```python
from build123d import *

# Parameters (mm, degrees)
BOSS_EXTRUDE1_START = -3
SKETCH2_R           = 9.461289508
BOSS_EXTRUDE1_DEPTH = 3
SKETCH3_R           = 2.54
BOSS_EXTRUDE2_DEPTH = 6
SKETCH4_R           = 2.54
CUT_EXTRUDE1_DEPTH  = 3


with BuildPart() as part:
    # Sketch1 → Revolve1 (revolve)
    with BuildSketch(Plane.XY, mode=Mode.PRIVATE) as revolve1_sk:
        with BuildLine():
            Line((-3, 3), (-3, 0))
            Line((-3, 0), (3, 0))
            ThreePointArc((3, 0), (3.464967985, 1.122532015), (4.5875, 1.5875))
            Line((4.5875, 1.5875), (3, 3))
            Line((3, 3), (0, 3))
            Line((0, 3), (-3, 3))
        make_face()
    revolve(revolve1_sk.sketch.rotate(Axis((-35.1, 18.916479231, 0), (0, -1, 0)), 180), axis=Axis((-35.1, 18.916479231, 0), (0, -1, 0)))

    # Sketch2 → Boss-Extrude1 (add)
    with BuildSketch(Plane(origin=(0, 3, 0), x_dir=(1, 0, 0), z_dir=(0, 1, 0)).offset(BOSS_EXTRUDE1_START)):
        with BuildLine():
            Line((-45.417440708, 11.981122365), (-56.04641595, 24.324014037))
            ThreePointArc((-56.04641595, 24.324014037), (-51.15, 27.799415461), (-45.692006103, 30.302135349))
            Line((-45.692006103, 30.302135349), (-40.31723598, 14.925726938))
            ThreePointArc((-40.31723598, 14.925726938), (-35.1, 15.811289508), (-29.88276402, 14.925726938))
            Line((-29.88276402, 14.925726938), (-24.507993897, 30.302135349))
            ThreePointArc((-24.507993897, 30.302135349), (-19.05, 27.799415461), (-14.15358405, 24.324014037))
            Line((-14.15358405, 24.324014037), (-24.782559292, 11.981122365))
            ThreePointArc((-24.782559292, 11.981122365), (-21.40702162, 7.905644754), (-19.565323312, 2.944604573))
            Line((-19.565323312, 2.944604573), (-3.561577947, 5.978121313))
            ThreePointArc((-3.561577947, 5.978121313), (-3, 0), (-3.561577947, -5.978121313))
            Line((-3.561577947, -5.978121313), (-19.565323312, -2.944604573))
            ThreePointArc((-19.565323312, -2.944604573), (-21.40702162, -7.905644754), (-24.782559292, -11.981122365))
            Line((-24.782559292, -11.981122365), (-14.15358405, -24.324014037))
            ThreePointArc((-14.15358405, -24.324014037), (-19.05, -27.799415461), (-24.507993897, -30.302135349))
            Line((-24.507993897, -30.302135349), (-29.88276402, -14.925726938))
            ThreePointArc((-29.88276402, -14.925726938), (-35.1, -15.811289508), (-40.31723598, -14.925726938))
            Line((-40.31723598, -14.925726938), (-45.692006103, -30.302135349))
            ThreePointArc((-45.692006103, -30.302135349), (-51.15, -27.799415461), (-56.04641595, -24.324014037))
            Line((-56.04641595, -24.324014037), (-45.417440708, -11.981122365))
            ThreePointArc((-45.417440708, -11.981122365), (-48.79297838, -7.905644754), (-50.634676688, -2.944604573))
            Line((-50.634676688, -2.944604573), (-66.638422053, -5.978121313))
            ThreePointArc((-66.638422053, -5.978121313), (-67.2, 0), (-66.638422053, 5.978121313))
            Line((-66.638422053, 5.978121313), (-50.634676688, 2.944604573))
            ThreePointArc((-50.634676688, 2.944604573), (-48.79297838, 7.905644754), (-45.417440708, 11.981122365))
        make_face()
        with Locations(Location((-35.1, 0, 0), (0, 0, 180))):
            Circle(SKETCH2_R, mode=Mode.SUBTRACT)
    extrude(amount=BOSS_EXTRUDE1_DEPTH)

    # Sketch3 → Boss-Extrude2 (add)
    with BuildSketch(Plane(origin=(0, 3, 0), x_dir=(1, 0, 0), z_dir=(0, 1, 0))):
        with Locations(Location((-46.983837426, 20.583410211, 0), (0, 0, 180))):
            Circle(SKETCH3_R)
        with Locations(Location((-11.332325148, 0, 0), (0, 0, 180))):
            Circle(SKETCH3_R)
        with Locations(Location((-46.983837426, -20.583410211, 0), (0, 0, 180))):
            Circle(SKETCH3_R)
    extrude(amount=-BOSS_EXTRUDE2_DEPTH)

    # Sketch4 → Cut-Extrude1 (cut)
    with BuildSketch(Plane(origin=(0, 3, 0), x_dir=(1, 0, 0), z_dir=(0, 1, 0))):
        with Locations(Location((-23.216162574, 20.583410211, 0), (0, 0, 180))):
            Circle(SKETCH4_R)
        with Locations(Location((-23.216162574, -20.583410211, 0), (0, 0, 180))):
            Circle(SKETCH4_R)
        with Locations(Location((-58.867674852, 0, 0), (0, 0, 180))):
            Circle(SKETCH4_R)
    extrude(amount=-CUT_EXTRUDE1_DEPTH, mode=Mode.SUBTRACT)


solid = part.part
```
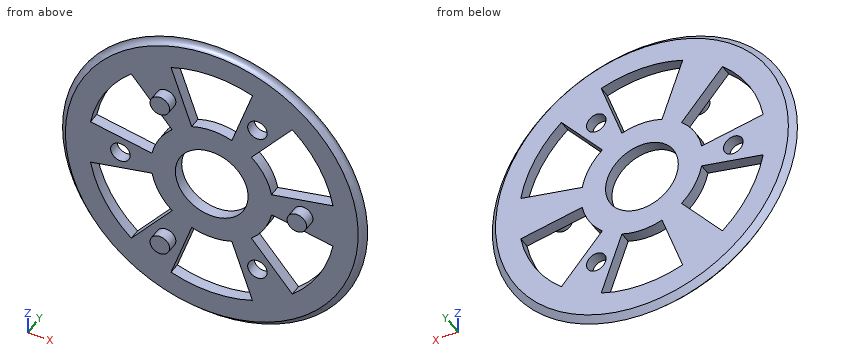
Check sheet for the modelled part. Datum: model origin and axes. Units: mm. Round coordinates to 2 decimals unless told otherwise and drop trailing zeros. Order: outer loops, then holes, each group sorted by start corner. A loop starts at its lowest first (then second) coordinate and runs counter-clockwise, first axis right, second up.
1) Section check B-B (x = -35.1). Record the boundary of the cut face in (y, z) (1 decimal).
2) Scan lines: line 1 (Z direction, x = -53.5, y = 2.2); line 2 (X direction, y = 0.15, z = 19.5); line 3 (Z direction, x = -9.5, y = 0.45). Record each from-to range of solid material in increasing order.
3) Section check D-D (x = -17). Give the number of separate pieces and of enclosed holes in the cut face, and give its area (3 significant figures).
4) Go/stop test with flat-tipped pins: pin 1 Ø2 at (y, z) = (-0.5, 14) entering from +X; pin 2 Ø1 at (x, y) = (-39, 1.5) entering from +Z; pin 3 Ø10 at (x, z) = (-10.5, 31) entering from -Y. Record where each tip stops, or that it passes through.
5) Section check A-A (z = 0). Record the boundary of the cut face in (x, y) (1 decimal).
6) Section check C-C (y = -1.1). Record the boundary of the cut face in (x, z).
Result:
1. outline: (0, -38.1) arc R1.6 cw to (1.6, -39.7) - (3, -38.1) - (3, -32.1) - (0, -32.1) - close; (0, -15.8) - (3, -15.8) - (3, -9.5) - (0, -9.5) - close; (0, 9.5) - (3, 9.5) - (3, 15.8) - (0, 15.8) - close; (0, 32.1) - (3, 32.1) - (3, 38.1) - (1.6, 39.7) arc R1.6 cw to (0, 38.1) - close
2. line 1: z = -34.39 to -21.37, -3.49 to 3.49, 21.37 to 34.39
2. line 2: x = -67.84 to -60.6, -51.89 to -41.92, -28.28 to -25.51, -20.92 to -18.31, -9.6 to -2.36
2. line 3: z = -28.31 to -19.37, -4.85 to 4.85, 19.37 to 28.31
3. separate pieces: 3
3. enclosed holes: 0
3. area: 99.4 mm2
4. pin 1: stops at x = 0.66
4. pin 2: stops at z = 39.54
4. pin 3: stops at y = 0
5. outline: (-74.8, 1.6) arc R1.6 cw to (-73.2, 0) - (-61.4, 0) - (-61.4, 3) - (-73.2, 3) - close; (-56.3, 0) - (-44.6, 0) - (-44.6, 3) - (-56.3, 3) - close; (-25.6, 0) - (-13.9, 0) - (-13.9, -3) - (-8.8, -3) - (-8.8, 0) - (3, 0) arc R1.6 cw to (4.6, 1.6) - (3, 3) - (-25.6, 3) - close
6. outline: circle Ø5.08 at (-46.98, -20.58); circle Ø5.08 at (-46.98, 20.58); circle Ø5.08 at (-11.33, 0)
